Autodesk Inventor part; units mm, degrees
ref_plane "YZ Plane" through (0, 0, 0) normal (1, 0, 0) x (0, 1, 0)
ref_plane "XZ Plane" through (0, 0, 0) normal (0, 1, 0) x (-1, 0, 0)
ref_plane "XY Plane" through (0, 0, 0) normal (0, 0, 1) x (1, 0, 0)
sketch "Sketch1" plane through (0, 0, 0) normal (0, 1, 0) x (-1, 0, 0)
  line L0 (7.366, 6.1452) -> (7.366, -23.8548)
  line L1 (7.366, -23.8548) -> (0, -23.8548)
  line L2 (6.096, -8.0476) -> (6.096, -9.0212)
  line L3 (0, 0.4868) -> (0, 3.5348)
  line L4 (6.096, 3.5348) -> (6.096, -8.0476)
  line L5 (0, -9.0212) -> (0, -11.8152)
  line L6 (6.096, -12.0692) -> (6.096, -9.0212)
  line L7 (6.096, 3.5348) -> (0, 0.4868)
  line L8 (6.096, -12.0692) -> (0, -9.0212)
  line L9 (0, -23.8548) -> (0, -9.0212)
  line L10 (0, 0.4868) -> (0, 16.3788)
  line L11 (6.096, 13.3308) -> (6.096, 16.3788)
  line L12 (6.096, 13.3308) -> (0, 16.3788)
  line L13 (6.096, 28.9348) -> (6.096, 17.3524)
  line L14 (6.096, 28.9348) -> (0, 25.8868)
  line L15 (6.096, 17.3524) -> (6.096, 16.3788)
  line L16 (6.096, 38.7308) -> (6.096, 41.7788)
  line L17 (6.096, 38.7308) -> (0, 41.7788)
  line L18 (6.096, 54.3348) -> (6.096, 42.7524)
  line L19 (6.096, 54.3348) -> (0, 51.2868)
  line L20 (6.096, 42.7524) -> (6.096, 41.7788)
  line L21 (6.096, 64.1308) -> (6.096, 67.1788)
  line L22 (6.096, 64.1308) -> (0, 67.1788)
  line L23 (6.096, 79.7348) -> (6.096, 68.1524)
  line L24 (6.096, 79.7348) -> (0, 76.6868)
  line L25 (6.096, 68.1524) -> (6.096, 67.1788)
  line L26 (7.366, 6.1452) -> (7.366, 91.622)
  line L27 (7.366, 91.622) -> (0, 91.622)
  line L28 (0, 25.8868) -> (0, 41.7788)
  line L29 (0, 51.2868) -> (0, 67.1788)
  line L30 (0, 76.6868) -> (0, 91.622)
  line L31 (6.096, -4.2672) -> (4.0009, -4.2672) construction
  point P0 (0, 0)
  dimension "d0" = 7.366
  dimension "d8" = 9.508
  dimension "d10" = 3.048
  dimension "d11" = 3.048
  dimension "d12" = 6.096
  dimension "d17" = 25.4
  dimension "d24" = 11.7856
  dimension "d67" = 115.4768
  dimension "d70" = 23.8548
  dimension "d71" = 4.754
extrude "MultipleTeeth" add sketch "Sketch1" along normal blind 19.05
sketch "Sketch2" plane through (0, 0, 0) normal (0, -1, 0) x (1, 0, 0)
  line L0 (0, 0.4868) -> (-6.096, 3.5348) construction
  line L1 (-6.096, 3.5348) -> (-6.096, -12.0692) construction
  line L2 (-6.096, -12.0692) -> (0, -9.0212) construction
  line L3 (0, 16.3788) -> (0, 0.4868)
  line L4 (0, 0.4868) -> (-6.096, 3.5348)
  line L5 (-6.096, -12.0692) -> (0, -9.0212)
  line L6 (-6.096, 3.5348) -> (-6.096, -12.0692)
  line L7 (-6.096, -12.0692) -> (-6.096, 3.5348)
  line L8 (0, -9.0212) -> (-6.096, -12.0692)
  line L9 (-7.366, -23.8548) -> (-7.366, 91.622)
  line L10 (-7.366, -59.508) -> (-7.366, -32.8548)
  line L11 (-7.366, -23.8548) -> (0, -23.8548)
  line L12 (-7.366, 91.622) -> (0, 91.622)
  line L13 (-7.366, -55.8503) -> (-7.366, -40.458) construction
  line L14 (0, -43.0234) -> (0, -59.508) construction
  line L15 (-6.096, -62.0648) -> (0, -62.0648) construction
  line L16 (0, -32.8548) -> (0, -37.6258)
  line L17 (0, -49.9828) -> (0, -62.0648)
  line L18 (0, -62.0648) -> (0, -59.508)
  line L19 (0, -32.8548) -> (-7.366, -32.8548) construction
  line L20 (0, -51.9048) -> (-7.366, -51.9048) construction
  line L21 (0, -42.3798) -> (-7.366, -42.3798) construction
  line L22 (-6.096, -12.0692) -> (-6.096, -62.0648) construction
  line L23 (0, -37.6258) -> (-6.096, -34.5778)
  line L24 (-6.096, -50.1818) -> (-6.096, -34.5778)
  line L25 (0, -47.1338) -> (-6.096, -50.1818)
  line L26 (0, -9.0212) -> (0, -23.8548)
  line L27 (0, -23.8548) -> (0, -32.8548)
  line L28 (-7.366, -32.8548) -> (-7.366, -23.8548)
  line L29 (0, -49.9828) -> (0, -47.1338)
  line L30 (0, -62.0648) -> (-7.366, -62.0648)
  line L31 (-7.366, -62.0648) -> (-7.366, -59.508)
  point P0 (0, 0)
  dimension "d25" = 115.4768
  dimension "d33" = 9
  dimension "d34" = 19.05
  dimension "d36" = 9.525
  dimension "d38" = 10.16
extrude "LongTooth" add sketch "Sketch2" against normal blind 100.2792
sketch "Sketch3" plane through (0, 19.05, 0) normal (0, 1, 0) x (1, 0, 0)
  line L0 (-6.096, -3.5348) -> (-6.096, 12.0692) construction
  line L1 (0, 23.8548) -> (-7.366, 23.8548)
  line L2 (-7.366, -91.622) -> (0, -91.622)
  line L3 (-7.366, 23.8548) -> (-6.096, 23.8548)
  line L4 (-6.096, 23.8548) -> (-6.096, -91.622)
  line L5 (-6.096, -91.622) -> (-7.366, -91.622)
  line L6 (-7.366, -91.622) -> (-7.366, 23.8548)
  point P0 (0, 0)
extrude "ThinPlate" add sketch "Sketch3" along normal up to surface (81.2292 mm away)
sketch "Sketch4" plane through (0, 0, 0) normal (0, -1, 0) x (1, 0, 0)
  line L0 (-6.096, 91.622) -> (0, 91.622)
  line L1 (-7.366, 91.622) -> (-7.366, -62.0648)
  line L2 (0, 91.622) -> (-7.366, 91.622)
  line L3 (-7.366, 91.622) -> (-7.366, -62.0648)
  line L4 (-7.366, -62.0648) -> (0, -62.0648)
  line L5 (0, -62.0648) -> (0, 91.622)
  point P0 (0, 0)
extrude "Extrusion4" add sketch "Sketch4" along normal blind 5.08
ref_plane "Work Plane1" through (-15.892, 0, 8.4328) normal (0, 0, 1) x (0, 1, 0)
sketch "Sketch6" plane through (0, 19.05, 16.3788) normal (1, 0, 0) x (0, 0, -1)
  circle A0 centre (71.4586, -8.89) radius 1.9304
  line L0 (78.4436, -24.13) -> (78.4436, 81.2292)
  line L1 (78.4436, -24.13) -> (-75.2432, -24.13)
  circle A1 centre (58.7586, -8.89) radius 1.9304
  circle A2 centre (46.0586, -8.89) radius 1.9304
  circle A3 centre (71.4586, 3.81) radius 1.9304
  circle A4 centre (58.7586, 3.81) radius 1.9304
  circle A5 centre (46.0586, 3.81) radius 1.9304
  circle A6 centre (71.4586, 16.51) radius 1.9304
  circle A7 centre (58.7586, 16.51) radius 1.9304
  circle A8 centre (46.0586, 16.51) radius 1.9304
  circle A9 centre (71.4586, 29.21) radius 1.9304
  circle A10 centre (58.7586, 29.21) radius 1.9304
  circle A11 centre (46.0586, 29.21) radius 1.9304
  circle A12 centre (71.4586, 41.91) radius 1.9304
  circle A13 centre (58.7586, 41.91) radius 1.9304
  circle A14 centre (46.0586, 41.91) radius 1.9304
  circle A15 centre (71.4586, 54.61) radius 1.9304
  circle A16 centre (58.7586, 54.61) radius 1.9304
  circle A17 centre (46.0586, 54.61) radius 1.9304
  circle A18 centre (71.4586, 67.31) radius 1.9304
  circle A19 centre (58.7586, 67.31) radius 1.9304
  circle A20 centre (46.0586, 67.31) radius 1.9304
  circle A21 centre (33.3586, -8.89) radius 1.9304
  circle A22 centre (33.3586, 3.81) radius 1.9304
  circle A23 centre (33.3586, 16.51) radius 1.9304
  circle A24 centre (33.3586, 29.21) radius 1.9304
  circle A25 centre (33.3586, 41.91) radius 1.9304
  circle A26 centre (33.3586, 54.61) radius 1.9304
  circle A27 centre (33.3586, 67.31) radius 1.9304
  circle A28 centre (20.6586, -8.89) radius 1.9304
  circle A29 centre (20.6586, 3.81) radius 1.9304
  circle A30 centre (20.6586, 16.51) radius 1.9304
  circle A31 centre (20.6586, 29.21) radius 1.9304
  circle A32 centre (20.6586, 41.91) radius 1.9304
  circle A33 centre (20.6586, 54.61) radius 1.9304
  circle A34 centre (20.6586, 67.31) radius 1.9304
  circle A35 centre (7.9586, -8.89) radius 1.9304
  circle A36 centre (7.9586, 3.81) radius 1.9304
  circle A37 centre (7.9586, 16.51) radius 1.9304
  circle A38 centre (7.9586, 29.21) radius 1.9304
  circle A39 centre (7.9586, 41.91) radius 1.9304
  circle A40 centre (7.9586, 54.61) radius 1.9304
  circle A41 centre (7.9586, 67.31) radius 1.9304
  circle A42 centre (-4.7414, -8.89) radius 1.9304
  circle A43 centre (-4.7414, 3.81) radius 1.9304
  circle A44 centre (-4.7414, 16.51) radius 1.9304
  circle A45 centre (-4.7414, 29.21) radius 1.9304
  circle A46 centre (-4.7414, 41.91) radius 1.9304
  circle A47 centre (-4.7414, 54.61) radius 1.9304
  circle A48 centre (-4.7414, 67.31) radius 1.9304
  circle A49 centre (-17.4414, -8.89) radius 1.9304
  circle A50 centre (-17.4414, 3.81) radius 1.9304
  circle A51 centre (-17.4414, 16.51) radius 1.9304
  circle A52 centre (-17.4414, 29.21) radius 1.9304
  circle A53 centre (-17.4414, 41.91) radius 1.9304
  circle A54 centre (-17.4414, 54.61) radius 1.9304
  circle A55 centre (-17.4414, 67.31) radius 1.9304
  circle A56 centre (-30.1414, -8.89) radius 1.9304
  circle A57 centre (-30.1414, 3.81) radius 1.9304
  circle A58 centre (-30.1414, 16.51) radius 1.9304
  circle A59 centre (-30.1414, 29.21) radius 1.9304
  circle A60 centre (-30.1414, 41.91) radius 1.9304
  circle A61 centre (-30.1414, 54.61) radius 1.9304
  circle A62 centre (-30.1414, 67.31) radius 1.9304
  circle A63 centre (-42.8414, -8.89) radius 1.9304
  circle A64 centre (-42.8414, 3.81) radius 1.9304
  circle A65 centre (-42.8414, 16.51) radius 1.9304
  circle A66 centre (-42.8414, 29.21) radius 1.9304
  circle A67 centre (-42.8414, 41.91) radius 1.9304
  circle A68 centre (-42.8414, 54.61) radius 1.9304
  circle A69 centre (-42.8414, 67.31) radius 1.9304
  circle A70 centre (-55.5414, -8.89) radius 1.9304
  circle A71 centre (-55.5414, 3.81) radius 1.9304
  circle A72 centre (-55.5414, 16.51) radius 1.9304
  circle A73 centre (-55.5414, 29.21) radius 1.9304
  circle A74 centre (-55.5414, 41.91) radius 1.9304
  circle A75 centre (-55.5414, 54.61) radius 1.9304
  circle A76 centre (-55.5414, 67.31) radius 1.9304
  circle A77 centre (-68.2414, -8.89) radius 1.9304
  circle A78 centre (-68.2414, 3.81) radius 1.9304
  circle A79 centre (-68.2414, 16.51) radius 1.9304
  circle A80 centre (-68.2414, 29.21) radius 1.9304
  circle A81 centre (-68.2414, 41.91) radius 1.9304
  circle A82 centre (-68.2414, 54.61) radius 1.9304
  circle A83 centre (-68.2414, 67.31) radius 1.9304
  point P0 (16.3788, -19.05)
  dimension "d56" = 3.8608
  dimension "d57" = 6.985
  dimension "d58" = 15.24
  dimension "d61" = 12.7
  dimension "d64" = 12.7
extrude "Extrusion5" cut sketch "Sketch6" against normal through all contours A0 | A2 | A6 | A8 | A12 | A14 | A18 | A20 | A21 | A23 | A25 | A27 | A35 | A37 | A39 | A41 | A49 | A51 | A53 | A55 | A63 | A65 | A67 | A69 | A77 | A79 | A81 | A83
sketch "Sketch7" plane through (0, 19.05, 16.3788) normal (1, 0, 0) x (0, 0, -1)
  circle A0 centre (-68.2414, -8.89) radius 1.9304
  circle A1 centre (-68.2414, -8.89) radius 4.445
  circle A2 centre (-42.8414, -8.89) radius 1.9304
  circle A3 centre (-42.8414, -8.89) radius 4.445
  circle A4 centre (-17.4414, -8.89) radius 1.9304
  circle A5 centre (-17.4414, -8.89) radius 4.445
  circle A6 centre (7.9586, -8.89) radius 1.9304
  circle A7 centre (7.9586, -8.89) radius 4.445
  circle A8 centre (33.3586, -8.89) radius 1.9304
  circle A9 centre (33.3586, -8.89) radius 4.445
  circle A10 centre (46.0586, -8.89) radius 1.9304
  circle A11 centre (46.0586, -8.89) radius 4.445
  circle A12 centre (71.4586, -8.89) radius 1.9304
  circle A13 centre (71.4586, -8.89) radius 4.445
  circle A14 centre (46.0586, 16.51) radius 1.9304
  circle A15 centre (46.0586, 16.51) radius 4.445
  circle A16 centre (71.4586, 16.51) radius 1.9304
  circle A17 centre (71.4586, 16.51) radius 4.445
  circle A18 centre (46.0586, 41.91) radius 1.9304
  circle A19 centre (46.0586, 41.91) radius 4.445
  circle A20 centre (71.4586, 41.91) radius 1.9304
  circle A21 centre (71.4586, 41.91) radius 4.445
  circle A22 centre (46.0586, 67.31) radius 1.9304
  circle A23 centre (46.0586, 67.31) radius 4.445
  circle A24 centre (71.4586, 67.31) radius 4.445
  point P0 (16.3788, -19.05)
  dimension "d74" = 8.89
  dimension "d75" = 8.89
  dimension "d76" = 8.89
  dimension "d77" = 8.89
  dimension "d78" = 8.89
  dimension "d79" = 8.89
  dimension "d80" = 8.89
  dimension "d81" = 8.89
  dimension "d82" = 8.89
  dimension "d83" = 8.89
  dimension "d84" = 8.89
  dimension "d85" = 8.89
  dimension "d86" = 8.89
extrude "Extrusion6" cut sketch "Sketch7" against normal blind 2.8194 contours A0 | A1 | A2 | A3 | A4 | A5 | A6 | A7 | A8 | A9 | A10 | A11 | A12 | A13 | A14 | A15 | A16 | A17 | A18 | A19 | A20 | A21 | A22 | A23 | A24
sketch "Sketch8" plane through (-7.366, 100.2792, -62.0648) normal (-1, 0, 0) x (0, 0, 1)
  circle A0 centre (138.9603, -20.6021) radius 7.5
  arc A1 (150.2591, -17.4048) -> (150.2591, -23.7995) centre (150.2591, -20.6021) ccw
  line L0 (151.6317, -23.7995) -> (150.2591, -23.7995)
  line L1 (150.2591, -17.4048) -> (151.6317, -17.4048)
  arc A2 (151.6317, -23.7995) -> (151.6317, -17.4048) centre (151.6317, -20.6021) ccw
  circle A3 centre (122.9454, -84.6021) radius 2.286 construction
  circle A4 centre (106.9454, -36.6021) radius 4
  circle A5 centre (106.9454, -4.6021) radius 4
  circle A6 centre (26.9454, -52.6021) radius 4 construction
  circle A7 centre (26.9454, -84.6021) radius 4 construction
  circle A8 centre (-5.0694, -68.6021) radius 7.5 construction
  circle A9 centre (-69.565, -9.819) radius 1.7 construction
  point P0 (62.0648, -100.2792)
extrude "Extrusion7" cut sketch "Sketch8" against normal blind 25.4
equation "\"d11\" = d10"
equation "\"d71\" = 0.5 * d8"
equation "\"d36\" = 0.5 * d34"
properties part number "Lift mount receiver left for metal drive train"
Design review of the part built by this model. Coordinates are the model's own, in mm. A direction names the side the tool comes from. Give positions to 0.01 mm unless a question says otherwise; leave off trailing zeros. Write each loop counter-clockwise with the first axis right and the second up, starting at its lowest first coordinate (ties: lowest second). Pieces come first, ordered by that corner, then holes. Notation, with made-up numbers: (20, -37.5) -> (66, -37.5) arc R19 cw to (66, -21.5) -> close; hole circle Ø1 at (77.5, 71). An arc over 180 degrees is marked (long way). Answer in a Markdown table with one row per item.
(1) Consider section C-C (z = -6.5). State the section outline as (x, y) points, then the cut area to 3 significant figures.
Results:
| item | result |
|---|---|
| outline | (-7.37, -5.08) -> (0, -5.08) -> (0, 0) -> (-6.1, 0) -> (-6.1, 100.28) -> (-7.37, 100.28) -> close |
| area | 165 mm2 |
(2) Consider section A-A (y = 42). State the section outline as (x, z) points.
Results:
| item | result |
|---|---|
| outline | (-7.37, -62.06) -> (0, -62.06) -> (0, -47.13) -> (-6.1, -50.18) -> (-6.1, -34.58) -> (0, -37.63) -> (0, -23.85) -> (-6.1, -23.85) -> (-6.1, 91.62) -> (-7.37, 91.62) -> close |
(3) Consider section D-D (y = 10.16). Count the separate pieces of the cut face and the enclosed holes in it, then the cut area to 3 significant figures.
Results:
| item | result |
|---|---|
| separate pieces | 8 |
| enclosed holes | 0 |
| area | 451 mm2 |
(4) Consider section B-B (z = 45). State the section outline as (x, y) points.
Results:
| item | result |
|---|---|
| outline | (-7.37, -5.08) -> (0, -5.08) -> (0, 0) -> (-6.1, 0) -> (-6.1, 59.68) -> (-7.37, 59.68) -> close; (-7.37, 67.68) -> (-6.1, 67.68) -> (-6.1, 91.68) -> (-7.37, 91.68) -> close; (-7.37, 99.68) -> (-6.1, 99.68) -> (-6.1, 100.28) -> (-7.37, 100.28) -> close |
(5) For faces 1 (the flat face through (-3, 19.05, 84)), 2 (the flat face through (-2.819, 8, 7)), 3 (the cylindrical face through (-6.722, 59.076, 8.839)), 4 (the flat face through (-3, 0, -42)), list the 3-axis set-ups (+Z, -Z, +X, -X, +Y, -Y) from which the entire face can be reached by the end or side of a thin tool; tool diameter is ignored.
Results:
| item | result |
|---|---|
| face 1 | +Z, +X, +Y |
| face 2 | +X |
| face 3 | +X, -X |
| face 4 | +Y |
(6) Clearance check with flat-ended pins moving along their axes: pin 1 (11.5 mm diameter, centred on y = 86.36, z = -55.08, fed in from -X); pin 2 (4.5 mm diameter, centred on y = 34.5, z = -30.5, fed in from +X); pin 3 (1 mm diameter, centred on x = -5, z = 59, fed in from +Y); pin 4 (3 mm diameter, centred on y = 58, z = -5, fed in from +X). State where each tip first meets the part, or that it passes through.
Results:
| item | result |
|---|---|
| pin 1 | x = -7.37 |
| pin 2 | x = -2.82 |
| pin 3 | y = 19.05 |
| pin 4 | x = -6.1 |
(7) To check wall thickness, follow probe 1 along Z at (x, y) = (-2.5, 18); probe 2 along Y at (x, z) = (-1, -53.5); probe 3 along Y at (x, z) = (-6.25, 46). State the ranges of each line that lie inside material, in increasing order.
Results:
| item | result |
|---|---|
| probe 1 | -62.06 to -48.38, -36.38 to -10.27, 1.74 to 15.13, 27.14 to 40.53, 52.54 to 65.93, 77.94 to 91.62 |
| probe 2 | -5.08 to 6.01, 14.31 to 31.41, 39.71 to 56.81, 65.11 to 82.21, 90.51 to 100.28 |
| probe 3 | -5.08 to 59.84, 67.52 to 91.84, 99.52 to 100.28 |
(8) Mouldability with a two-part tool opening along X and no side actions: class faces 5 (the flat face through (-3.091, 9.392, 40.233)), 6 (the flat face through (-2.819, 84, -56)), 7 (the cylindrical face through (-1.39, 62.3, -59.32)) as +X half, -X half, draft (parallel to the pull), parting line (faces both ways), or undercut.
Results:
| item | result |
|---|---|
| face 5 | undercut |
| face 6 | +X half |
| face 7 | draft |
